For this review, take the finished solid that the model builds, in its own axes (mm). A direction names the side the tool comes from. Give positions to 0.01 mm unless a question says otherwise; leave off trailing zeros. Loops run counter-clockwise (first coordinate to the right, second up) from the corner with the lowest first, then second, coordinate; pieces in that order, holes last.
```python
from build123d import *

# Parameters (mm, degrees)
POG_BIENIE_STO_KOWE_POD_M6_WKR_T_Z_BEM_D           = 6.6
POG_BIENIE_STO_KOWE_POD_M6_WKR_T_Z_BEM_DEPTH       = 30
POG_BIENIE_STO_KOWE_POD_M6_WKR_T_Z_BEM_CSINK_D     = 13.44
POG_BIENIE_STO_KOWE_POD_M6_WKR_T_Z_BEM_CSINK_ANGLE = 90
POG_BIENIE_STO_KOWE_POD_M6_WKR_T_Z_BEM_TIP         = 1.982840043


with BuildPart() as part:
    # Szkic2 → Obr_t1 (revolve)
    with BuildSketch(Plane(origin=(0, 0, 0), x_dir=(1, 0, 0), z_dir=(0, 1, 0)), mode=Mode.PRIVATE) as obr_t1_sk:
        Polygon((0, 0), (45, 0), (45, -4), (62.5, -4), (62.5, -8), (0, -8), align=None)
    revolve(obr_t1_sk.sketch.rotate(Axis((0, 0, 8), (0, 0, -1)), 180), axis=Axis((0, 0, 8), (0, 0, -1)))

    # Szkic1 → Wyci_cie-obr_t1 (revolve, cut)
    with BuildSketch(Plane(origin=(0, 0, 0), x_dir=(1, 0, 0), z_dir=(0, 1, 0)), mode=Mode.PRIVATE) as wyci_cie_obr_t1_sk:
        Polygon((0, 0), (18, 0), (18, -1), (25, -8), (0, -8), align=None)
    revolve(wyci_cie_obr_t1_sk.sketch.rotate(Axis((0, 0, 8), (0, 0, -1)), 180), axis=Axis((0, 0, 8), (0, 0, -1)), mode=Mode.SUBTRACT)

    # Pog_bienie sto_kowe pod M6 Wkr_t z _bem
    with Locations(Plane(origin=(-55, 0, 8), x_dir=(1, 0, 0), z_dir=(0, 0, 1))):
        with Locations((0, 0), (55, 55), (110, 0), (55, -55)):
            CounterSinkHole(POG_BIENIE_STO_KOWE_POD_M6_WKR_T_Z_BEM_D / 2, POG_BIENIE_STO_KOWE_POD_M6_WKR_T_Z_BEM_CSINK_D / 2, depth=POG_BIENIE_STO_KOWE_POD_M6_WKR_T_Z_BEM_DEPTH, counter_sink_angle=POG_BIENIE_STO_KOWE_POD_M6_WKR_T_Z_BEM_CSINK_ANGLE)
            with Locations((0, 0, -(POG_BIENIE_STO_KOWE_POD_M6_WKR_T_Z_BEM_DEPTH + POG_BIENIE_STO_KOWE_POD_M6_WKR_T_Z_BEM_TIP / 2))):  # 118° drill point
                Cone(0, POG_BIENIE_STO_KOWE_POD_M6_WKR_T_Z_BEM_D / 2, POG_BIENIE_STO_KOWE_POD_M6_WKR_T_Z_BEM_TIP, mode=Mode.SUBTRACT)


solid = part.part
```
Q1. For pin 1 Ø1.5 at (x, y) = (41, 5.5) entering from -Z; pin 2 Ø3 at (x, z) = (-21, 7) entering from -Y; pin 3 Ø7.5 at (x, y) = (0, -55) entering from -Z; pin 4 Ø5.5 at (x, y) = (-55, 0) entering from +Z, all flat-tipped, find the tip position at first contact; note any pin that passes through.
Answers:
pin 1: stops at z = 0
pin 2: stops at y = -59.38
pin 3: stops at z = 4
pin 4: passes through
Q2. Mouldability with a two-part tool opening along Y and no side actions: class faces 3 (the flat face through (1, -27, 8)), 4 (the cylindrical face through (62.44, 2.75, 6.03)), 5 (the cylindrical face through (58.3, 0.1, 4.3)) as +Y half, -Y half, draft (parallel to the pull), parting line (faces both ways), or undercut.
Answers:
face 3: draft
face 4: parting line
face 5: undercut
Q3. Machinability: for faces 1 (the cylindrical face through (-20.765, -39.923, 2.028)), 2 (the conical face through (51.69, 1.04, 4.75)), which of the approach directions +Z, -Z, +X, -X, +Y, -Y give a long, thin tool a straight path to every point of the face, cutting with its end or side? Answer none if there is none.
Answers:
face 1: -Z
face 2: +Z
Q4. Consider section A-A on x = 0. Give the boundary of the cut face in (y, z), plus the area to 3 significant figures.
Answers:
outline: (-62.5, 4) - (-58.3, 4) - (-58.3, 4.58) - (-61.72, 8) - (-62.5, 8) - close; (-51.7, 4) - (-45, 4) - (-45, 0) - (-18, 0) - (-18, 1) - (-25, 8) - (-48.28, 8) - (-51.7, 4.58) - close; (18, 0) - (45, 0) - (45, 4) - (51.7, 4) - (51.7, 4.58) - (48.28, 8) - (25, 8) - (18, 1) - close; (58.3, 4) - (62.5, 4) - (62.5, 8) - (61.72, 8) - (58.3, 4.58) - close
area: 447 mm2
Q5. Consider section C-C on z = 6. Give the boundary of the cut face in (x, y), plus the area to 3 significant figures.
Answers:
outline: circle Ø125 at (0, 0); hole circle Ø9.44 at (-55, 0); hole circle Ø46 at (0, 0); hole circle Ø9.44 at (0, -55); hole circle Ø9.44 at (0, 55); hole circle Ø9.44 at (55, 0)
area: 10,300 mm2
Q6. For probe 1 along Y at (x, z) = (0, 4.35); probe 2 along Y at (x, z) = (0, 4.4); probe 3 along Z at (x, y) = (24, -49), list the stretches that pass through material, from the lowest coordinate up.
Answers:
probe 1: y = -62.5 to -58.3, -51.7 to -21.35, 21.35 to 51.7, 58.3 to 62.5
probe 2: y = -62.5 to -58.3, -51.7 to -21.4, 21.4 to 51.7, 58.3 to 62.5
probe 3: z = 4 to 8
Q7. Consider section D-D on x = 55. Give the boundary of the cut face in (y, z), plus the area to 3 significant figures.
Answers:
outline: (-29.69, 4) - (-3.3, 4) - (-3.3, 4.58) - (-6.72, 8) - (-29.69, 8) - close; (3.3, 4) - (29.69, 4) - (29.69, 8) - (6.72, 8) - (3.3, 4.58) - close
area: 199 mm2
